Design review of the part built by this model. Coordinates are the model's own, in mm. Face numbers are marked on the shaded views. A direction names the side the tool comes from. Give positions to 0.01 mm unless a question says otherwise; leave off trailing zeros. Loops run counter-clockwise (first coordinate to the right, second up) from the corner with the lowest first, then second, coordinate; pieces in that order, holes last. Notation, with made-up numbers: (-4.75, 46) -> (12.25, 46) arc R21 cw to (12.25, 61) -> close; hole circle Ø8 at (-19, -13). An arc over 180 degrees is marked (long way). Use a Markdown table: item, result. Add a question column.
1. To check wall thickness, follow line 1 (Y direction, x = 0, z = -85.6); line 2 (Z direction, x = 9.5, y = 9.5) (3 decimals); line 3 (X direction, y = -27, z = -89). State the ranges of each line that lie inside material, in increasing order.
2. Add section A-A (z = -88.5). State the section outline as (x, y) points (1 decimal), and give its area (3 significant figures).
3. Add section B-B (x = 0). State the section outline as (y, z) points (1 decimal).
4. For the marked faces 5, 6, 7 and 8, list the 3-axis set-ups (+Z, -Z, +X, -X, +Y, -Y) from which the entire face can be reached by the end or side of a thin tool; tool diameter is ignored.
5. For pin 1 Ø5 at (y, z) = (23.5, -92) entering from -X; pin 2 Ø5.5 at (x, y) = (-2.5, -30.5) entering from -Z (3 decimals); pin 3 Ø10.5 at (x, y) = (7.5, -7.5) entering from +Z, all flat-tipped, find the tip position at first contact; note any pin that passes through.
6. Add section D-D (z = -84.75). State the section outline as (x, y) points (1 decimal).
7. Draft analysis for pull direction Y (two halves, no side actions). For the marked faces 1, 2, 3 and 4, state which applies: pulls with the +Y half, pulls with the -Y half, needs draft (parallel to the pull), parting line crosses it, or undercut.
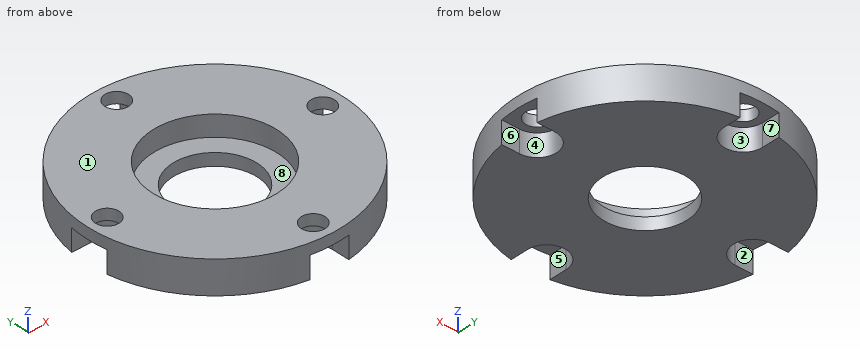
```python
from build123d import *

# Parameters (mm, degrees)
CBORE_FOR_1_4_SOCKET_HEAD_CAP_SCREW1_D           = 6.7564
CBORE_FOR_1_4_SOCKET_HEAD_CAP_SCREW1_CBORE_D     = 11.1125
CBORE_FOR_1_4_SOCKET_HEAD_CAP_SCREW1_CBORE_DEPTH = 6.35
CUT_EXTRUDE1_DEPTH                               = 6.35


with BuildPart() as part:
    # Cap → Endcap-Revolve (revolve)
    with BuildSketch(Plane(origin=(0, 0, 0), x_dir=(0, 0, -1), z_dir=(1, 0, 0)), mode=Mode.PRIVATE) as endcap_revolve_sk:
        Polygon((93.345, 12.065), (89.789, 12.065), (89.789, 17.78), (83.82, 17.78), (83.82, 36.5125), (93.345, 36.5125), align=None)
    revolve(endcap_revolve_sk.sketch.rotate(Axis((0, 0, -141.5522592), (0, 0, 1)), 90), axis=Axis((0, 0, -141.5522592), (0, 0, 1)))

    # CBORE for 1/4 Socket Head Cap Screw1 (through all)
    with Locations(Plane(origin=(0, 0, -93.345), x_dir=(-1, 0, 0), z_dir=(0, 0, -1))):
        with Locations((0, 30.95752), (30.95752, 0), (0, -30.95752), (-30.95752, 0)):
            CounterBoreHole(CBORE_FOR_1_4_SOCKET_HEAD_CAP_SCREW1_D / 2, CBORE_FOR_1_4_SOCKET_HEAD_CAP_SCREW1_CBORE_D / 2, CBORE_FOR_1_4_SOCKET_HEAD_CAP_SCREW1_CBORE_DEPTH)

    # Bolt-Clearance → Cut-Extrude1 (cut)
    with BuildSketch(Plane(origin=(0, 0, -93.345), x_dir=(-1, 0, 0), z_dir=(0, 0, -1))):
        Polygon((5.55625, 30.95752), (5.55625, 37.30752), (-5.55625, 37.30752), (-5.55625, 30.95752), (0, 30.95752), align=None)
        Polygon((30.95752, 0), (30.95752, 5.55625), (37.30752, 5.55625), (37.30752, -5.55625), (30.95752, -5.55625), align=None)
        Polygon((0, -30.95752), (5.55625, -30.95752), (5.55625, -37.30752), (-5.55625, -37.30752), (-5.55625, -30.95752), align=None)
        Polygon((-30.95752, 0), (-30.95752, -5.55625), (-37.30752, -5.55625), (-37.30752, 5.55625), (-30.95752, 5.55625), align=None)
    extrude(amount=-CUT_EXTRUDE1_DEPTH, mode=Mode.SUBTRACT)


solid = part.part
```
Taken from the geometry:
| question | item | result |
|---|---|---|
| 1 | line 1 | y = -36.51 to -34.34, -27.58 to -17.78, 17.78 to 27.58, 34.34 to 36.51 |
| 1 | line 2 | z = -93.345 to -89.789 |
| 1 | line 3 | x = -24.58 to -3.9, 3.9 to 24.58 |
| 2 | outline | (-36.1, -5.6) arc R36.5 ccw to (-5.6, -36.1) -> (-5.6, -31) arc R5.6 cw to (5.6, -31) -> (5.6, -36.1) arc R36.5 ccw to (36.1, -5.6) -> (31, -5.6) arc R5.6 cw to (31, 5.6) -> (36.1, 5.6) arc R36.5 ccw to (5.6, 36.1) -> (5.6, 31) arc R5.6 cw to (-5.6, 31) -> (-5.6, 36.1) arc R36.5 ccw to (-36.1, 5.6) -> (-31, 5.6) arc R5.6 cw to (-31, -5.6) -> close; hole circle Ø35.6 at (0, 0) |
| 2 | area | 2,760 mm^2 |
| 3 | outline | (-36.5, -87) -> (-34.3, -87) -> (-34.3, -83.8) -> (-36.5, -83.8) -> close; (-27.6, -87) -> (-25.4, -87) -> (-25.4, -93.3) -> (-12.1, -93.3) -> (-12.1, -89.8) -> (-17.8, -89.8) -> (-17.8, -83.8) -> (-27.6, -83.8) -> close; (12.1, -93.3) -> (25.4, -93.3) -> (25.4, -87) -> (27.6, -87) -> (27.6, -83.8) -> (17.8, -83.8) -> (17.8, -89.8) -> (12.1, -89.8) -> close; (34.3, -87) -> (36.5, -87) -> (36.5, -83.8) -> (34.3, -83.8) -> close |
| 4 | face 5 | -Z, -Y |
| 4 | face 6 | -Z, +X |
| 4 | face 7 | -Z, +Y |
| 4 | face 8 | +Z |
| 5 | pin 1 | stops at x = -29.87 |
| 5 | pin 2 | stops at z = -86.995 |
| 5 | pin 3 | stops at z = -89.79 |
| 6 | outline | circle Ø73 at (0, 0); hole circle Ø6.8 at (-31, 0); hole circle Ø35.6 at (0, 0); hole circle Ø6.8 at (0, -31); hole circle Ø6.8 at (0, 31); hole circle Ø6.8 at (31, 0) |
| 7 | face 1 | needs draft |
| 7 | face 2 | undercut |
| 7 | face 3 | pulls with the +Y half |
| 7 | face 4 | undercut |
